Build history of the part. All positions in model axes, mm. Round coordinates to 2 decimals unless told otherwise and drop trailing zeros. Loops run counter-clockwise (first coordinate to the right, second up) from the corner with the lowest first, then second, coordinate; pieces in that order, holes last. Notation, with made-up numbers: M 2,12 L 30,12 A21 cw 30,38 Z; hole C -0.5,-24 d5. An arc over 180 degrees is marked long. One line per item, written item: value.
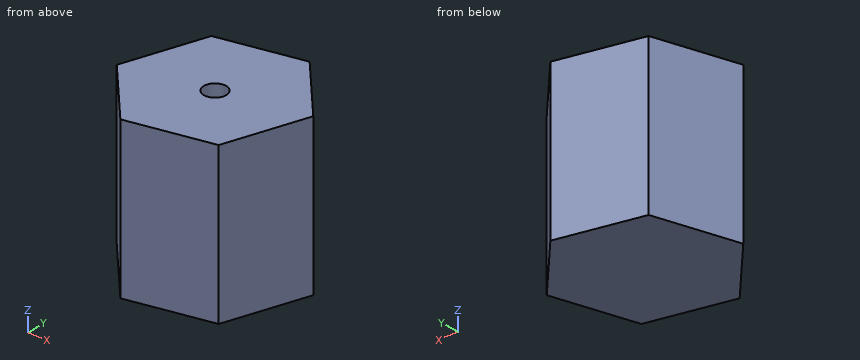
Autodesk Fusion 360 part; units mm, degrees
sketch "Sketch1" plane through (0, 0, 0) normal (0, 0, 1) x (1, 0, 0)
  line L0 (2.5647, -2.804) -> (3.7107, 0.819)
  line L1 (3.7107, 0.819) -> (1.146, 3.6231)
  line L2 (1.146, 3.6231) -> (-2.5647, 2.804)
  line L3 (-2.5647, 2.804) -> (-3.7107, -0.819)
  line L4 (-3.7107, -0.819) -> (-1.146, -3.6231)
  line L5 (-1.146, -3.6231) -> (2.5647, -2.804)
  dimension "d1" = 3.8
extrude "Extrude1" add sketch "Sketch1" along normal blind 7
sketch "Sketch2" plane through (0, 0, 7) normal (0, 0, 1) x (-1, 0, 0)
  line L0 (1.146, 3.6231) -> (-2.5647, 2.804)
  line L1 (-2.5647, 2.804) -> (-3.7107, -0.819)
  line L2 (-3.7107, -0.819) -> (-1.146, -3.6231)
  line L3 (-1.146, -3.6231) -> (2.5647, -2.804)
  line L4 (2.5647, -2.804) -> (3.7107, 0.819)
  line L5 (3.7107, 0.819) -> (1.146, 3.6231)
  circle A0 centre (0, 0) radius 0.5
  dimension "d6" = 1
extrude "Extrude3" cut sketch "Sketch2" against normal blind 1 contours A0
equation "d1 = polygon_side"
equation "d2 = polygon_height"
equation "polygon_side = 3.8 mm"
equation "polygon_height = 7 mm"
equation "d6 = nail_radius * 2"
equation "nail_radius = 0.5 mm"
equation "nail_depth = 1 mm"
Item 1: Wall check: line 1 along X through (y, z) = (0, 6.45); line 2 along Y through (x, z) = (0, 6.45); line 3 along Y through (x, z) = (-2.25, 1.75). Give the ranges that are in metal, low to high.
Check values:
line 1: x = -3.45 to -0.5, 0.5 to 3.45
line 2: y = -3.37 to -0.5, 0.5 to 3.37
line 3: y = -2.42 to 2.87
Item 2: Drop flat-ended pins along their axis: P1, Ø1, axis at y = 2.5, z = 5, coming from the -X side; P2, Ø3, axis at x = 1.5, z = 3, coming from the +Y side; P3, Ø3, axis at x = 3, z = 2, coming from the -Y side; P4, Ø0.8, axis at x = 0, y = 0, coming from the +Z side. Give the stop position or say it passes through.
Check values:
P1: stops at x = -2.82
P2: stops at y = 3.62
P3: stops at y = -3.04
P4: stops at z = 6
Item 3: Slice it at C-C, the plane y = 0. Give the cut face in (x, z).
Check values:
outline: M -3.45,0 L 3.45,0 L 3.45,7 L 0.5,7 L 0.5,6 L -0.5,6 L -0.5,7 L -3.45,7 Z
Item 4: Slice it at A-A, the plane z = 2. Give the cut face in (x, y).
Check values:
outline: M -3.71,-0.82 L -1.15,-3.62 L 2.56,-2.8 L 3.71,0.82 L 1.15,3.62 L -2.56,2.8 Z
Item 5: Slice it at B-B, the plane x = 0. Give the cut face in (y, z), and give its area (3 significant figures).
Check values:
outline: M -3.37,0 L 3.37,0 L 3.37,7 L 0.5,7 L 0.5,6 L -0.5,6 L -0.5,7 L -3.37,7 Z
area: 46.2 mm2
Item 6: Slice it at D-D, the plane x = -2. Give the cut face in (y, z).
Check values:
outline: M -2.69,0 L 2.93,0 L 2.93,7 L -2.69,7 Z
